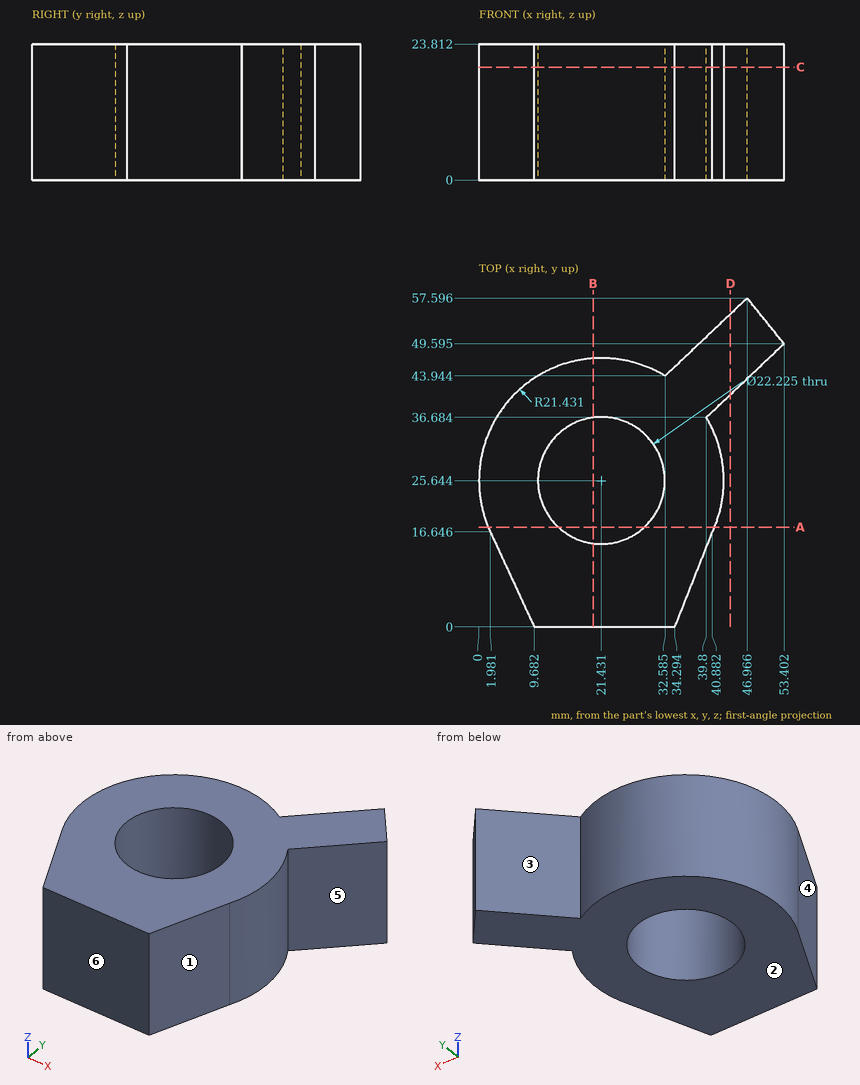
Answer from the drawing. Dimensions are ordinates in mm from the lowest x, y and z of the part. A direction names the side the tool comes from. Coordinates: 2 decimals unless noted, no trailing zeros. Write each loop counter-clockwise with the first axis right and the second up, starting at its lowest first coordinate (ties: lowest second). Pieces come first, ordered by that corner, then holes. Notation, with made-up numbers: (47.5, 88) - (91.5, 88) arc R26 ccw to (91.5, 116) - close; hole circle Ø10 at (65, -29). An arc over 180 degrees is marked (long way). Return JSON: item names as keys, results as strings. Group by question number.
Q1. Flat-ended cylindrical pins translate along their axes: pin 1 Ø12 at (x, z) = (5.5, 6) entering from +Y (1 decimal); pin 2 Ø10 at (y, z) = (44.5, 10.5) entering from -X; pin 3 Ø8 at (y, z) = (45.5, 14.5) entering from -X; pin 4 Ø8 at (x, y) = (8.5, 40) entering from -Z. Find the tip coordinate at first contact, or state that the pin passes through.
Q2. For a pull along X with two mould halves and no side action, classify the marked faces 1, 2, 3 and 4 as +X half, -X half, draft (parallel to the pull), parting line (faces both ways), or undercut.
Q3. Which of the six approach directions +Z, -Z, +X, -X, +Y, -Y give full straight-line access (tool end or side, diameter ignored) to the marked faces 5 and 6?
Q4. The part is cut by section B-B on x = 20. Write down the section's boundary in (y, z) (1 decimal).
Q5. The part is cut by section C-C on z = 19.75. Write down the section's boundary in (x, y) (1 decimal), and give its area (3 significant figures).
Q6. The part is cut by section D-D on x = 44. Write down the section's boundary in (y, z).
Q7. Find the intervals of material crossed by line 1 along X through (y, z) = (24, 14.5); line 2 along Y through (x, z) = (23, 21.5) (1 decimal); line 3 along Y through (x, z) = (27.5, 9) (1 decimal), in increasing order. Write a range as [from, to].
Q8. The part is cut by section A-A on y = 17.5. Write down the section's boundary in (x, z) (1 decimal).
Evaluation:
{
 "1": {"pin 1": "stops at y = 44.6", "pin 2": "stops at x = 5.08", "pin 3": "stops at x = 7.01", "pin 4": "stops at z = 0"},
 "2": {"face 1": "+X half", "face 2": "draft", "face 3": "undercut", "face 4": "-X half"},
 "3": {"face 5": "+Z, -Z, +X", "face 6": "+Z, -Z, +X, -X, -Y"},
 "4": {"outline": "(0, 0) - (14.6, 0) - (14.6, 23.8) - (0, 23.8) - close; (36.7, 0) - (47, 0) - (47, 23.8) - (36.7, 23.8) - close"},
 "5": {"outline": "(2, 16.6) - (9.7, 0) - (34.3, 0) - (40.9, 16.6) arc R21.4 ccw to (39.8, 36.7) - (53.4, 49.6) - (47, 57.6) - (32.6, 43.9) arc R21.4 ccw to start; hole circle Ø22.2 at (21.4, 25.6)", "area": "1,430 mm2"},
 "6": {"outline": "(40.67, 0) - (54.78, 0) - (54.78, 23.81) - (40.67, 23.81) - close"},
 "7": {"line 1": "x = [0.06, 10.44], [32.42, 42.8]", "line 2": "y = [0, 14.6], [36.6, 47]", "line 3": "y = [0, 16.3], [35, 46.2]"},
 "8": {"outline": "(1.6, 0) - (13.9, 0) - (13.9, 23.8) - (1.6, 23.8) - close; (29, 0) - (41.3, 0) - (41.3, 23.8) - (29, 23.8) - close"}
}
